from build123d import *

# Parameters (mm, degrees)
SKETCH1_W               = 323
SKETCH1_H               = 45.34
BOSS_EXTRUDE1_DEPTH     = 3
SKETCH2_R               = 6
SKETCH2_R_2             = 2.4
SKETCH2_R_3             = 14.5
SKETCH2_R_4             = 1.5
SKETCH2_W               = 71
SKETCH2_H               = 24.5
SKETCH2_W_2             = 28
SKETCH2_H_2             = 31
CUT_EXTRUDE1_DEPTH      = 1
CUT_EXTRUDE1_DEPTH_BACK = 4


with BuildPart() as part:
    # Sketch1 → Boss-Extrude1 (new body)
    with BuildSketch(Plane.XY):
        Rectangle(SKETCH1_W, SKETCH1_H)
    extrude(amount=BOSS_EXTRUDE1_DEPTH)

    # Sketch2 → Cut-Extrude1 (cut, two sides)
    with BuildSketch(Plane.XY.offset(3)) as cut_extrude1_sk:
        with Locations((44, 0)):
            Circle(SKETCH2_R)
        with Locations((74, 0)):
            Circle(SKETCH2_R_2)
        with Locations((44, 15.67)):
            Circle(SKETCH2_R_2)
        with Locations((134, 0)):
            Circle(SKETCH2_R_2)
        with Locations((119, 0)):
            Circle(SKETCH2_R_2)
        with Locations((104, 0)):
            Circle(SKETCH2_R_2)
        with Locations((-39.75, 0)):
            Circle(SKETCH2_R_3)
        with Locations((-155.5, 16.55)):
            Circle(SKETCH2_R_4)
        with Locations((-155.5, -15.05)):
            Circle(SKETCH2_R_4)
        with Locations((155.5, -15.05)):
            Circle(SKETCH2_R_4)
        with Locations((155.5, 16.55)):
            Circle(SKETCH2_R_4)
        with Locations((-101, 0)):
            Rectangle(SKETCH2_W, SKETCH2_H)
        Rectangle(SKETCH2_W_2, SKETCH2_H_2)
    extrude(amount=CUT_EXTRUDE1_DEPTH, mode=Mode.SUBTRACT)
    extrude(cut_extrude1_sk.sketch, amount=-CUT_EXTRUDE1_DEPTH_BACK, mode=Mode.SUBTRACT)


solid = part.part
Could you check a few things on this model? Use its own coordinates, in mm. Round coordinates to 2 decimals unless told otherwise and drop trailing zeros. Order: outer loops, then holes, each group sorted by start corner. A loop starts at its lowest first (then second) coordinate and runs counter-clockwise, first axis right, second up.
Q1. I'm going to push a flat-ended pin straight in: P1, Ø3, axis at x = 119, y = 0, coming from the +Z side. Where does the tip first touch, or does it pass through?
Geometry says:
P1: passes through
Q2. Imagine slicing it at B-B, the plane z = 1.05. State how many separate pieces and enclosed holes the cut face has, then the cut area to 3 significant figures.
Geometry says:
separate pieces: 1
enclosed holes: 13
area: 11,100 mm2
Q3. Imagine slicing it at A-A, the plane x = -106. List the corners of the cut face in (y, z) for me.
Geometry says:
outline: (-22.67, 0) - (-12.25, 0) - (-12.25, 3) - (-22.67, 3) - close; (12.25, 0) - (22.67, 0) - (22.67, 3) - (12.25, 3) - close
Q4. Please list where these lines run through material, in increasing order: probe 1 along Y at (x, z) = (155.5, 2.1); probe 2 along Y at (x, z) = (-134, 1.3); probe 3 along Y at (x, z) = (74, 0.9).
Geometry says:
probe 1: y = -22.67 to -16.55, -13.55 to 15.05, 18.05 to 22.67
probe 2: y = -22.67 to -12.25, 12.25 to 22.67
probe 3: y = -22.67 to -2.4, 2.4 to 22.67
Q5. Thinking about a two-plate mould opening in X: for faces 1 (the face through (-51.26, -8.82, 1.52)), 2 (the face through (34, 0, 0)), which applies, released by +X, released by -X, zero draft, split by the parting line, or undercut?
Geometry says:
face 1: undercut
face 2: zero draft
